```python
from build123d import *

# Parameters (mm, degrees)
F0_R          = 1
F1_DEPTH      = 2
F1_DEPTH_BACK = 2
F3_R          = 0.85
F4_DEPTH      = 26.001
F5_R          = 1.5


with BuildPart() as f1:
    # F0 (on Top) → F1 (new body, two sides)
    with BuildSketch(Plane.XY) as f1_sk:
        with BuildLine():
            ThreePointArc((6.25, 0), (0, -6.25), (-6.25, 0))
            Line((-6.25, 0), (-6.25, 2.5))
            Line((-6.25, 2.5), (-13, 2.5))
            Line((-13, 2.5), (-13, -23.5))
            Line((-13, -23.5), (13, -23.5))
            Line((13, -23.5), (13, 2.5))
            Line((13, 2.5), (6.25, 2.5))
            Line((6.25, 2.5), (6.25, 0))
        make_face()
        with Locations((-10.5, -21)):
            Circle(F0_R, mode=Mode.SUBTRACT)
        with Locations((10.5, -21)):
            Circle(F0_R, mode=Mode.SUBTRACT)
        with Locations((-10.5, 0)):
            Circle(F0_R, mode=Mode.SUBTRACT)
        with Locations((10.5, 0)):
            Circle(F0_R, mode=Mode.SUBTRACT)
    extrude(amount=F1_DEPTH)
    extrude(f1_sk.sketch, amount=-F1_DEPTH_BACK)

    # F3 (on face) → F4 (cut, through all)
    with BuildSketch(Plane.YZ.offset(13)):
        with Locations((-10.5, 0)):
            Circle(F3_R)
        with Locations((-3, 0)):
            Circle(F3_R)
        with Locations((-18, 0)):
            Circle(F3_R)
    extrude(amount=-F4_DEPTH, mode=Mode.SUBTRACT)

    # F5
    f5_edges = [f1.edges().sort_by_distance(p)[0] for p in [
        (-13, 2.5, 0),
        (13, 2.5, 0),
        (6.25, 2.5, 0),
        (-6.25, 2.5, 0),
        (-13, -23.5, 0),
        (13, -23.5, 0),
    ]]
    fillet(f5_edges, radius=F5_R)


solid = f1.part
```
Geometry: final body of the model. Coordinates: model frame, mm. A direction names the side the tool comes from. Round coordinates to 2 decimals unless told otherwise and drop trailing zeros. Order: outer loops, then holes, each group sorted by start corner. A loop starts at its lowest first (then second) coordinate and runs counter-clockwise, first axis right, second up. Notation, with made-up numbers: (-23.75, 1.25) -> (6.25, 1.25) arc R12 cw to (6.25, 8.25) -> close; hole circle Ø8 at (-12, 0.5). An arc over 180 degrees is marked (long way). Use one line per item in the form item = value.
(1) Section B-B on z = 1.45. Return loops of the section in (x, y), and give its area (3 significant figures).
Results list:
outline = (-13, -22) arc R1.5 ccw to (-11.5, -23.5) -> (11.5, -23.5) arc R1.5 ccw to (13, -22) -> (13, 1) arc R1.5 ccw to (11.5, 2.5) -> (7.75, 2.5) arc R1.5 ccw to (6.25, 1) -> (6.25, 0) arc R6.25 cw to (-6.25, 0) -> (-6.25, 1) arc R1.5 ccw to (-7.75, 2.5) -> (-11.5, 2.5) arc R1.5 ccw to (-13, 1) -> close; hole circle Ø2 at (-10.5, -21); hole circle Ø2 at (-10.5, 0); hole circle Ø2 at (10.5, -21); hole circle Ø2 at (10.5, 0)
area = 568 mm^2
(2) Ray query, probe 1 along Z at (x, y) = (-11.25, -3); probe 2 along Y at (x, z) = (-10.5, -0.6); probe 3 along Y at (x, z) = (-3, -0.4). Return the intervals inside material, ascending. Write a range as [from, to].
Results list:
probe_1 = [-2, -0.85], [0.85, 2]
probe_2 = [-23.5, -22], [-20, -18.6], [-17.4, -11.1], [-9.9, -3.6], [-2.4, -1], [1, 2.5]
probe_3 = [-23.5, -18.75], [-17.25, -11.25], [-9.75, -5.48]
(3) Section A-A on x = -10.5. Return loops of the section in (y, z), and give its area (3 significant figures).
Results list:
outline = (-23.5, -2) -> (-22, -2) -> (-22, 2) -> (-23.5, 2) -> close; (-20, -2) -> (-1, -2) -> (-1, 2) -> (-20, 2) -> close; (1, -2) -> (2.5, -2) -> (2.5, 2) -> (1, 2) -> close; hole circle Ø1.7 at (-18, 0); hole circle Ø1.7 at (-10.5, 0); hole circle Ø1.7 at (-3, 0)
area = 81.2 mm^2
(4) Access query for faces 5 (the face through (6.68, 2.05, -0.03)), 6 (the face through (12.55, 2.07, -0.03)). Directions: +Z, -Z, +X, -X, +Y, -Y. A direction counts if a zero-diameter tool reaches every point of the face in a straight line with its end or side. Return the directions, or none.
Results list:
face_5 = +Z, -Z, +Y
face_6 = +Z, -Z, +X, +Y
(5) First-contact query: pin 1 Ø1 at (y, z) = (-3, 0) entering from +X. Flat tip, straight axial feed; report the tip coordinate or a pass-through.
Results list:
pin_1 = through
(6) Section D-D on y = -17.75. Return loops of the section in (x, z), and give its area (3 significant figures).
Results list:
outline = (-13, -2) -> (13, -2) -> (13, -0.81) -> (-13, -0.81) -> close; (-13, 0.81) -> (13, 0.81) -> (13, 2) -> (-13, 2) -> close
area = 61.8 mm^2
(7) Draft query along Y for faces 1 (the face through (0.182, -9.715, -0.326)), 2 (the face through (-12.57, -23.05, 0.03)), 3 (the face through (0.18, -18.67, -0.52)), 4 (the face through (-6.68, 2.05, 0.03)). Return one class per face: pulls with the +Y half, pulls with the -Y half, needs draft (parallel to the pull), parting line crosses it, or undercut.
Results list:
face_1 = undercut
face_2 = pulls with the -Y half
face_3 = undercut
face_4 = pulls with the +Y half
(8) Section C-C on y = -21. Return loops of the section in (x, z), and give its area (3 significant figures).
Results list:
outline = (-13, -2) -> (-11.5, -2) -> (-11.5, 2) -> (-13, 2) -> close; (-9.5, -2) -> (9.5, -2) -> (9.5, 2) -> (-9.5, 2) -> close; (11.5, -2) -> (13, -2) -> (13, 2) -> (11.5, 2) -> close
area = 88.0 mm^2
